from build123d import *

# Parameters (mm, degrees)
F0_W          = 240.03
F0_H          = 12.7
F1_DEPTH      = 6.35
F1_DEPTH_BACK = 6.35
F2_R          = 13.97
F3_DEPTH      = 17.78
F5_D          = 3.81
F7_D          = 3.81


with BuildPart() as f1:
    # F0 (on Front) → F1 (new body, two sides)
    with BuildSketch(Plane.XZ) as f1_sk:
        with Locations((-120.015, 6.35)):
            Rectangle(F0_W, F0_H)
    extrude(amount=F1_DEPTH)
    extrude(f1_sk.sketch, amount=-F1_DEPTH_BACK)

    # F2 (on face) → F3 (join)
    with BuildSketch(Plane(origin=(0, 0, 0), x_dir=(1, 0, 0), z_dir=(0, 0, -1))):
        Circle(F2_R)
    extrude(amount=-F3_DEPTH)

    # F5 (through all)
    with Locations(Plane.XY.offset(12.7)):
        with Locations((-233.68, 0), (-198.755, 0)):
            Hole(F5_D / 2)

    # F7 (through all)
    with Locations(Plane.XY.offset(17.78)):
        with Locations((-8.169546, 8.169546), (8.169546, 8.169546), (8.169546, -8.169546), (-8.169546, -8.169546)):
            Hole(F7_D / 2)


solid = f1.part
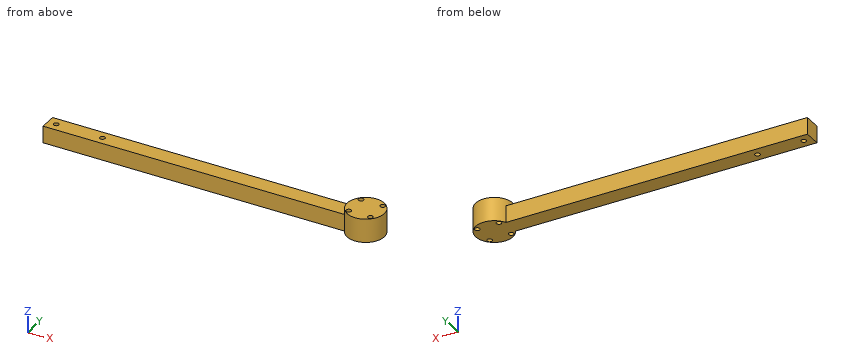
Work out the finished part from the listing and answer in its coordinate system (mm). Coordinates: 2 decimals unless noted, no trailing zeros. Loops run counter-clockwise (first coordinate to the right, second up) from the corner with the lowest first, then second, coordinate; pieces in that order, holes last. Notation, with made-up numbers: (83.25, 54.5) -> (124.25, 54.5) arc R18 ccw to (124.25, 85.5) -> close; hole circle Ø10 at (-5, -2). An arc over 180 degrees is marked (long way). Write each question's results on one line, items separated by ' | '. Start each with the question number.
1) Find section B-B on y = 4. Determine the outline of the cut face in (x, z), then the cut area to 3 significant figures.
2) Find section A-A on z = 3.5. Determine the outline of the cut face in (x, y) (3 decimals).
3) Consider line 1 along X through (y, z) = (-8, 12); line 2 along X through (y, z) = (-9.5, 15.5); line 3 along Y through (x, z) = (-109.5, 12.5). Determine where each line is inside the solid, lowest interval first.
4) Find section C-C on x = -140. Determine the outline of the cut face in (y, z), then the cut area to 3 significant figures.
5) Flat-ended cylindrical pins translate along their axes: P1, Ø4.5, axis at x = -8.17, y = -8.17, coming from the -Z side; P2, Ø4, axis at x = -103.5, z = 4.5, coming from the -Y side; P3, Ø4, axis at x = -152.5, z = 3.5, coming from the +Y side; P4, Ø6, axis at y = 5, z = 7, coming from the +X side. Find the tip coordinate at first contact, or state that the pin passes through.
6) Find section D-D on z = 15. Determine the outline of the cut face in (x, y) (3 decimals).
Response values:
1) outline: (-240.03, 0) -> (13.39, 0) -> (13.39, 17.78) -> (-13.39, 17.78) -> (-13.39, 12.7) -> (-240.03, 12.7) -> close | area: 3,350 mm^2
2) outline: (-240.03, -6.35) -> (-12.443, -6.35) arc R13.97 ccw (long way) to (-12.443, 6.35) -> (-240.03, 6.35) -> close; hole circle Ø3.81 at (-233.68, 0); hole circle Ø3.81 at (-198.755, 0); hole circle Ø3.81 at (-8.17, -8.17); hole circle Ø3.81 at (-8.17, 8.17); hole circle Ø3.81 at (8.17, -8.17); hole circle Ø3.81 at (8.17, 8.17)
3) line 1: x = -11.45 to -10.07, -6.27 to 6.27, 10.07 to 11.45 | line 2: x = -10.24 to -9.53, -6.81 to 6.81, 9.53 to 10.24 | line 3: y = -6.35 to 6.35
4) outline: (-6.35, 0) -> (6.35, 0) -> (6.35, 12.7) -> (-6.35, 12.7) -> close | area: 161 mm^2
5) P1: stops at z = 0 | P2: stops at y = -6.35 | P3: stops at y = 6.35 | P4: stops at x = 13.83
6) outline: circle Ø27.94 at (0, 0); hole circle Ø3.81 at (-8.17, -8.17); hole circle Ø3.81 at (-8.17, 8.17); hole circle Ø3.81 at (8.17, -8.17); hole circle Ø3.81 at (8.17, 8.17)
